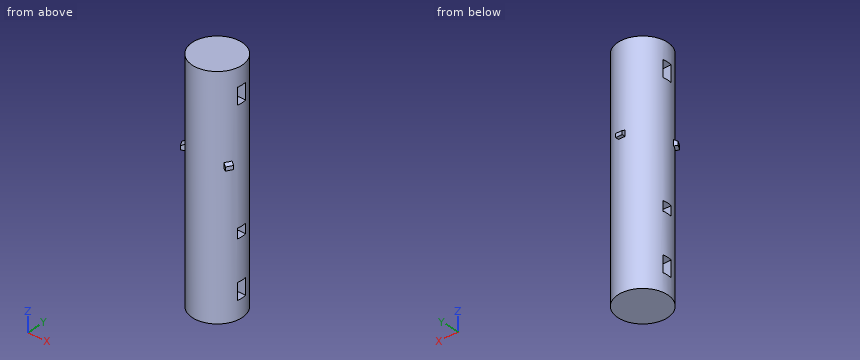
from build123d import *

# Parameters (mm, degrees)
SKETCH1_R               = 3.8
BOSS_EXTRUDE1_DEPTH     = 35.3
SKETCH3_W               = 2.5
SKETCH3_H               = 0.75
CUT_EXTRUDE2_DEPTH      = 36.706722056
CUT_EXTRUDE3_DEPTH      = 36.706722056
CUT_EXTRUDE3_DEPTH_BACK = 36.706722056
SKETCH6_W               = 1.5
SKETCH6_H               = 1.5
BOSS_EXTRUDE2_START     = -0.5
BOSS_EXTRUDE2_DEPTH     = 1
CIRPATTERN1_COUNT       = 3


# Read off the part's stored shape, not the designer's step: Boss-Extrude2
with BuildPart() as part:
    # Sketch1 → Boss-Extrude1 (new body)
    with BuildSketch(Plane.XY):
        Circle(SKETCH1_R)
    extrude(amount=BOSS_EXTRUDE1_DEPTH)

    # Sketch3 → Cut-Extrude2 (cut, symmetric)
    with BuildSketch(Plane(origin=(0, 0, 0), x_dir=(0, 0, -1), z_dir=(1, 0, 0))):
        with Locations((-31.3, -0.375)):
            Rectangle(SKETCH3_W, SKETCH3_H)
        with Locations((-31.3, 0.375)):
            Rectangle(SKETCH3_W, SKETCH3_H)
    cut_extrude2 = extrude(amount=CUT_EXTRUDE2_DEPTH, both=True, mode=Mode.SUBTRACT)

    # Mirror1: Cut-Extrude2 across plane
    add(cut_extrude2.mirror(Plane.XY.offset(17.65)), mode=Mode.SUBTRACT)

    # Sketch6 → Cut-Extrude3 (cut, two sides: drawn at the far end of the back side and taken through both)
    with BuildSketch(Plane(origin=(0, 0, 0), x_dir=(0, 0, -1), z_dir=(1, 0, 0)).offset(-CUT_EXTRUDE3_DEPTH_BACK)):
        with Locations((-12.1, 0)):
            Rectangle(SKETCH6_W, SKETCH6_H)
    extrude(amount=CUT_EXTRUDE3_DEPTH + CUT_EXTRUDE3_DEPTH_BACK, mode=Mode.SUBTRACT)

    # Boss-Extrude2 outline → Boss-Extrude2 (add)
    with BuildSketch(Plane(origin=(0, 0, 0), x_dir=(0, 0, -1), z_dir=(1, 0, 0)).offset(BOSS_EXTRUDE2_START)):
        Polygon((-22.227350269, 4.3), (-22.804700538, 3.3), (-21.65, 3.3), (-21.65, 4.3), align=None)
    boss_extrude2 = extrude(amount=BOSS_EXTRUDE2_DEPTH)

    # CirPattern1: Boss-Extrude2 ×3 about axis
    cirpattern1_axis = Axis((0, 0, 0), (0, 0, 1))
    for i in range(1, CIRPATTERN1_COUNT):
        add(boss_extrude2.rotate(cirpattern1_axis, i * 360 / CIRPATTERN1_COUNT))


solid = part.part
Geometry check sheet. Reference: the model listing, model coordinates, mm. Round coordinates to 2 decimals unless told otherwise and drop trailing zeros. Order: outer loops, then holes, each group sorted by start corner. A loop starts at its lowest first (then second) coordinate and runs counter-clockwise, first axis right, second up. Notation, with made-up numbers: (-39.5, -35.75) -> (-15.5, -35.75) arc R17 cw to (-15.5, -23.75) -> close; hole circle Ø11 at (49.25, 64). An arc over 180 degrees is marked (long way). Use one line per item in the form item = value.
1. Go/stop test with flat-tipped pins: pin 1 (2.5 mm diameter, centred on x = 0, z = 31.5, fed in from +Y); pin 2 (1.5 mm diameter, centred on x = -1.5, z = 18.5, fed in from +Y); pin 3 (1 mm diameter, centred on y = 2.5, z = 4.5, fed in from +X). Record where each tip stops, or that it passes through.
Working result:
pin_1 = 3.8
pin_2 = 3.73
pin_3 = 3.23
2. Cross-section at A-A, the plane y = 0. Enter the section's corners in (x, z).
Working result:
outline = (-3.8, 0) -> (3.8, 0) -> (3.8, 2.75) -> (-3.8, 2.75) -> close; (-3.8, 5.25) -> (3.8, 5.25) -> (3.8, 11.35) -> (-3.8, 11.35) -> close; (-3.8, 12.85) -> (3.8, 12.85) -> (3.8, 30.05) -> (-3.8, 30.05) -> close; (-3.8, 32.55) -> (3.8, 32.55) -> (3.8, 35.3) -> (-3.8, 35.3) -> close
3. Cross-section at D-D, the plane z = 10. Enter the section's corners in (x, y), plus the area to 3 significant figures.
Working result:
outline = circle Ø7.6 at (0, 0)
area = 45.4 mm^2
4. Cross-section at C-C, the plane x = 0. Enter the section's corners in (y, z), plus the area to 3 significant figures.
Working result:
outline = (-3.8, 0) -> (3.8, 0) -> (3.8, 21.65) -> (4.3, 21.65) -> (4.3, 22.23) -> (3.8, 22.52) -> (3.8, 35.3) -> (-3.8, 35.3) -> close; hole (-0.75, 2.75) -> (0.75, 2.75) -> (0.75, 5.25) -> (-0.75, 5.25) -> close; hole (-0.75, 11.35) -> (0.75, 11.35) -> (0.75, 12.85) -> (-0.75, 12.85) -> close; hole (-0.75, 30.05) -> (0.75, 30.05) -> (0.75, 32.55) -> (-0.75, 32.55) -> close
area = 259 mm^2
5. Scan lines: line 1 along Z through (x, y) = (1.25, -0.25); line 2 along X through (y, z) = (2.5, 3); line 3 along Y through (x, z) = (1, 4). Record each from-to range of solid material in increasing order. Write a range as from..to.
Working result:
line_1 = 0..2.75, 5.25..11.35, 12.85..30.05, 32.55..35.3
line_2 = -2.86..2.86
line_3 = -3.67..-0.75, 0.75..3.67
6. Cross-section at B-B, the plane z = 4. Enter the section's corners in (x, y), plus the area to 3 significant figures.
Working result:
outline = (-3.73, -0.75) arc R3.8 ccw to (3.73, -0.75) -> close; (-3.73, 0.75) -> (3.73, 0.75) arc R3.8 ccw to start
area = 34.0 mm^2
